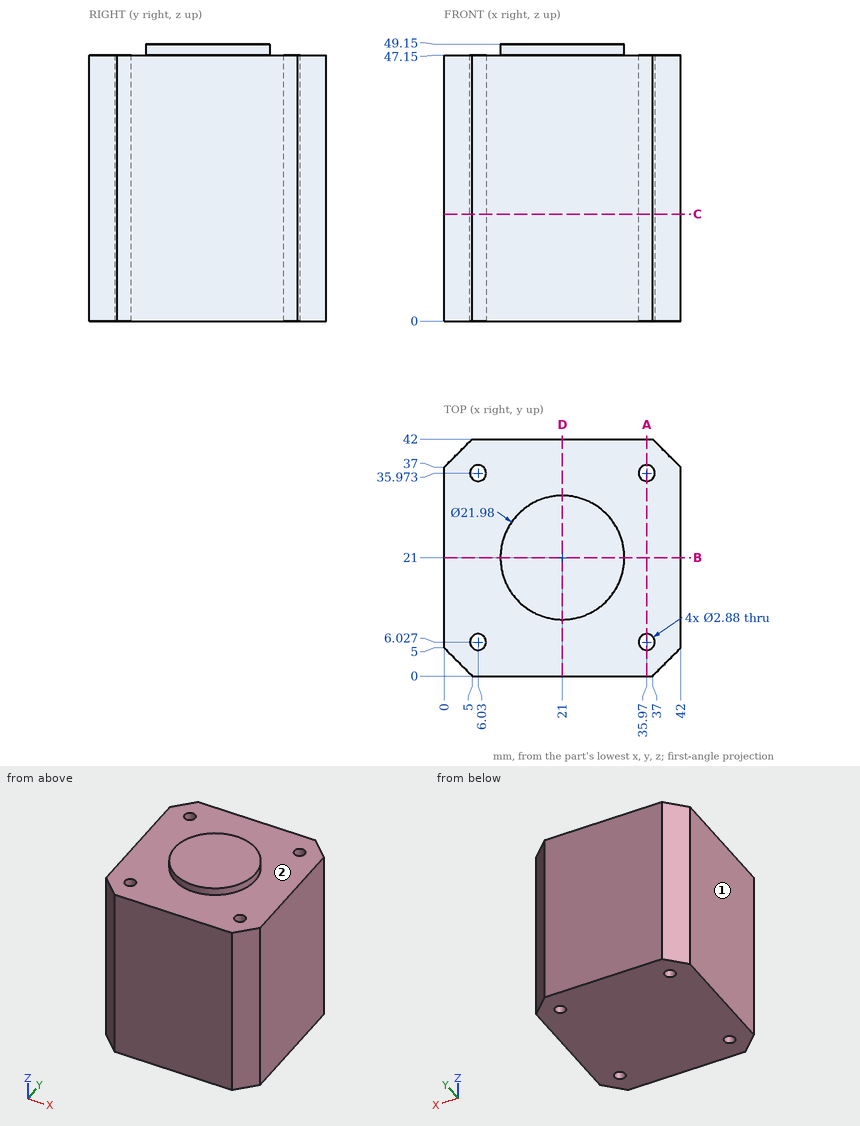
Part print with two shaded views. Sizes in mm from the minimum x, y, z corner. A direction names the side the tool comes from. Round coordinates to 2 decimals unless told otherwise and drop trailing zeros. Loops run counter-clockwise (first coordinate to the right, second up) from the corner with the lowest first, then second, coordinate; pieces in that order, holes last. Notation, with made-up numbers: M -21.5,81.25 L 3.5,81.25 A20 cw 3.5,85.25 Z; hole C 1.25,20 d4. An arc over 180 degrees is marked long. Put each result on its own line as item: value. Start each with the question number.
Item 1: Drop flat-ended pins along their axis: P1, Ø2.5, axis at x = 6.03, y = 35.97, coming from the +Z side; P2, Ø3.5, axis at x = 6.03, y = 6.03, coming from the +Z side. Give the stop position or say it passes through.
Item 2: Cut at B-B (y = 21). List the corners of the cut face in (x, z), then the cut area to 3 significant figures.
Item 3: 3-axis set-ups, long thin cutter, end or side, ignore diameter. For the marked faces 1 and 2: which of +Z, -Z, +X, -X, +Y, -Y reach the whole face in a straight line?
Item 4: Cut at C-C (z = 19). List the corners of the cut face in (x, y).
Item 5: Drill centre lines: line 1 along Y through (x, z) = (6.03, 33.5); line 2 along Y through (x, z) = (5, 20). Where is each one in solid material? Low to high.
Item 6: Cut at A-A (x = 35.97). List the corners of the cut face in (y, z).
Answer block:
1. P1: through
1. P2: z = 47.15
2. outline: M 0,0 L 42,0 L 42,47.15 L 31.99,47.15 L 31.99,49.15 L 10.01,49.15 L 10.01,47.15 L 0,47.15 Z
2. area: 2,020 mm2
3. face 1: +Z, -Z, -X, +Y, -Y
3. face 2: +Z
4. outline: M 0,5 L 5,0 L 37,0 L 42,5 L 42,37 L 37,42 L 5,42 L 0,37 Z; hole C 6.03,6.03 d2.88; hole C 6.03,35.97 d2.88; hole C 35.97,6.03 d2.88; hole C 35.97,35.97 d2.88
5. line 1: 0 to 4.59, 7.47 to 34.53, 37.41 to 42
5. line 2: 0 to 5.02, 7.03 to 34.97, 36.98 to 42
6. outline: M 0,0 L 4.59,0 L 4.59,47.15 L 0,47.15 Z; M 7.47,0 L 34.53,0 L 34.53,47.15 L 7.47,47.15 Z; M 37.41,0 L 42,0 L 42,47.15 L 37.41,47.15 Z
